For this review, take the finished solid that the model builds, in its own axes (mm). A direction names the side the tool comes from. Coordinates: 2 decimals unless noted, no trailing zeros. Write each loop counter-clockwise with the first axis right and the second up, starting at its lowest first coordinate (ties: lowest second). Pieces come first, ordered by that corner, then holes.
```python
from build123d import *

# Parameters (mm, degrees)
SKETCH031_W             = 10
SKETCH031_H             = 3
PAD005_DEPTH            = 25
SKETCH032_R             = 1.25
POCKET025_DEPTH         = 5
BOX002_W                = 10
BOX002_H                = 12
BOX002_DEPTH            = 3
SKETCH033_R             = 1.9
POCKET026_DEPTH         = 3.001
BODY004_ROLL_ANGLE      = -90
BODY004_PLACEMENT_ANGLE = 90


with BuildPart() as part:
    # Sketch031 → Pad005 (new body)
    with BuildSketch(Plane.XZ):
        with Locations((5, 1.5)):
            Rectangle(SKETCH031_W, SKETCH031_H)
    extrude(amount=PAD005_DEPTH)

    # Sketch032 (on Face3 of Pad005) → Pocket025 (cut)
    with BuildSketch(Plane(origin=(0, 0, 3), x_dir=(-1, 0, 0), z_dir=(0, 0, 1))):
        with Locations((-2.3, 18.9)):
            Circle(SKETCH032_R)
        with Locations((-2.3, 9.4)):
            Circle(SKETCH032_R)
    extrude(amount=-POCKET025_DEPTH, mode=Mode.SUBTRACT)

    # Box002 → Box002 (join)
    with BuildSketch(Plane(origin=(0, 0, 7.5), x_dir=(1, 0, 0), z_dir=(0, 1, 0))):
        with Locations((5, 6)):
            Rectangle(BOX002_W, BOX002_H)
    extrude(amount=BOX002_DEPTH)

    # Sketch033 → Pocket026 (cut, through all)
    with BuildSketch(Plane.XZ):
        with Locations((5, -2.25)):
            Circle(SKETCH033_R)
        with Locations((5, 5.25)):
            Circle(SKETCH033_R)
    extrude(amount=-POCKET026_DEPTH, mode=Mode.SUBTRACT)


with BuildPart() as part_1:
    # Body004 roll: moved
    add(part.part.rotate(Axis((0, 0, 0), (1, 0, 0)), BODY004_ROLL_ANGLE))


with BuildPart() as part_2:
    # Body004 placement: moved
    add(part_1.part.moved(Location((123.59503, 57.475552, 30.987237))).rotate(Axis((123.59503, 57.475552, 30.987237), (0, 0, 1)), BODY004_PLACEMENT_ANGLE))


solid = part_2.part
```
Q1. Add section A-A (x = 124.75). State the section outline as (y, z) points.
Ans:
outline: (57.48, 27.99) - (60.92, 27.99) - (60.92, 30.99) - (57.48, 30.99) - close; (64.03, 27.99) - (67.48, 27.99) - (67.48, 30.99) - (64.03, 30.99) - close
Q2. Add section D-D (x = 121.25). State the section outline as (y, z) points.
Ans:
outline: (57.48, 27.99) - (67.48, 27.99) - (67.48, 55.99) - (57.48, 55.99) - close; hole circle Ø2.5 at (59.78, 40.39); hole circle Ø2.5 at (59.78, 49.89)
Q3. For probe 1 along Y at (x, z) = (118.25, 30.75); probe 2 along X at (y, z) = (63, 30.75); probe 3 along Z at (x, y) = (117.25, 66), list the stretches that pass through material, from the lowest coordinate up.
Ans:
probe 1: y = 57.48 to 60.58, 64.37 to 67.48
probe 2: x = 116.1 to 116.52, 120.17 to 124.02, 127.67 to 128.1
probe 3: z = 27.99 to 30.99
Q4. Draft analysis for pull direction X (two halves, no side actions). For faces 4 (the cylindrical face through (120.03, 63.35, 29.51)), 5 (the cylindrical face through (127.7, 62.06, 29.51)), 6 (the flat face through (122, 62, 55.987)), 7 (the flat face through (120.595, 62, 43)), state which applies: +X half, -X half, draft (parallel to the pull), parting line (faces both ways), or undercut.
Ans:
face 4: undercut
face 5: undercut
face 6: draft
face 7: -X half
Q5. Clearance check with flat-ended pins moving along their axes: pin 1 Ø1 at (y, z) = (59.5, 37.5) entering from -X (3 decimals); pin 2 Ø3.5 at (x, y) = (118.5, 60.5) entering from +Z; pin 3 Ø1 at (y, z) = (59.5, 34.5) entering from +X (3 decimals). State where each tip first meets the part, or that it passes through.
Ans:
pin 1: stops at x = 120.595
pin 2: stops at z = 30.99
pin 3: stops at x = 123.595
Q6. Add section C-C (y = 65.75). State the section outline as (x, z) points, then the cut area to 3 significant figures.
Ans:
outline: (116.1, 27.99) - (128.1, 27.99) - (128.1, 30.99) - (123.6, 30.99) - (123.6, 55.99) - (120.6, 55.99) - (120.6, 30.99) - (116.1, 30.99) - close
area: 111 mm2
Q7. Add section B-B (y = 64). State the section outline as (x, z) points, then the cut area to 3 significant figures.
Ans:
outline: (116.1, 27.99) - (117.21, 27.99) - (117.21, 30.99) - (116.1, 30.99) - close; (119.48, 27.99) - (124.71, 27.99) - (124.71, 30.99) - (123.6, 30.99) - (123.6, 55.99) - (120.6, 55.99) - (120.6, 30.99) - (119.48, 30.99) - close; (126.98, 27.99) - (128.1, 27.99) - (128.1, 30.99) - (126.98, 30.99) - close
area: 97.4 mm2
Q8. Tool access review of faces 1 (the flat face through (120, 61, 30.987)), 2 (the flat face through (116.095, 62, 30)), 3 (the flat face through (123.595, 62, 43)): name each direction out of +Z, -Z, +X, -X, +Y, -Y from which nothing blocks a thin tool from reaching the whole face with its end or side.
Ans:
face 1: +Z, -X, +Y, -Y
face 2: +Z, -Z, -X, +Y, -Y
face 3: +Z, +X, +Y, -Y
